Verification items for the finished model (mm, model axes). Face numbers are marked on the shaded views. A direction names the side the tool comes from. Coordinates: 2 decimals unless noted, no trailing zeros. Order: outer loops, then holes, each group sorted by start corner. A loop starts at its lowest first (then second) coordinate and runs counter-clockwise, first axis right, second up. Notation, with made-up numbers: M 81.5,4 L 94.5,4 A25 cw 94.5,20 Z; hole C 42.25,-35.75 d6. An arc over 180 degrees is marked long. Return JSON: item names as keys, results as strings. Group by question number.
1. Gauge pin test, flat end, axial feed: pin 1 (8 mm diameter, centred on x = 25, z = 15, fed in from +Y). Record the tip position at first contact, or that the pin passes through.
2. Mould release check, pull along Z, two halves, no side actions. Record for the marked faces 1, 2, 3 and 4: +Z half, -Z half, draft (parallel to the pull), parting line (faces both ways), or undercut.
3. Section check D-D, the plane x = 33. Record the cut outline in (y, z), plus the area to 3 significant figures.
4. Section check A-A, the plane z = 15. Record the cut outline in (x, y), plus the area to 4 significant figures.
5. Section check C-C, the plane y = 124.5. Record the cut outline in (x, z).
6. Set-up check for the marked faces 5 and 6: record each of +Z, -Z, +X, -X, +Y, -Y from which the full face is reachable in a straight line by a thin tool's end or side.
7. Section check B-B, the plane y = 66. Record the cut outline in (x, z).
8. Material ranges on line 1 along X through (y, z) = (-1, 15); line 2 along Z through (x, y) = (12, 105); line 3 along Y through (x, z) = (4.5, 16.5), recorded low to high.
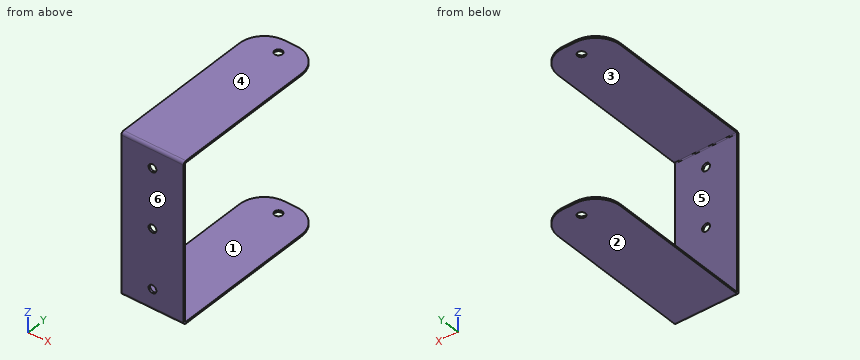
```python
from build123d import *

# Parameters (mm, degrees)
SKETCH1_W                    = 50
SKETCH1_H                    = 125
BASE_FLANGE1_DEPTH           = 1.5
EDGE_FLANGE1_STRIP_W         = 7.5
EDGE_FLANGE1_STRIP_H         = 1.5
EDGE_FLANGE1_STRIP_CUT_DEPTH = 50
EDGE_FLANGE1_DEPTH           = 50
SKETCH9_R                    = 3.15
CUT_EXTRUDE1_DEPTH           = 176
EDGE_FLANGE2_STRIP_W         = 7.5
EDGE_FLANGE2_STRIP_H         = 1.5
EDGE_FLANGE2_STRIP_CUT_DEPTH = 50
EDGE_FLANGE2_DEPTH           = 50
CUT_EXTRUDE2_START           = -10
SKETCH13_R                   = 3.15
CUT_EXTRUDE2_DEPTH           = 10
FILLET1_R                    = 20
SKETCH14_R                   = 3.15
CUT_EXTRUDE3_DEPTH           = 10


# Sheet-metal steps are written as plain solids
with BuildPart() as part:
    # Sketch1 → Base-Flange1 (new body)
    with BuildSketch(Plane(origin=(0, 0, 0), x_dir=(1, 0, 0), z_dir=(0, 1, 0))):
        with Locations((25, -62.5)):
            Rectangle(SKETCH1_W, SKETCH1_H)
    extrude(amount=-BASE_FLANGE1_DEPTH)

    # Edge-Flange1 strip (across the edge) → Edge-Flange1 strip cut (cut)
    with BuildSketch(Plane(origin=(0, 0, 125), x_dir=(0, 0, -1), z_dir=(1, 0, 0))):
        with Locations((-3, -0.75)):
            Rectangle(EDGE_FLANGE1_STRIP_W, EDGE_FLANGE1_STRIP_H)
    extrude(amount=EDGE_FLANGE1_STRIP_CUT_DEPTH, mode=Mode.SUBTRACT)

    # Edge-Flange1 section (across the edge) → Edge-Flange1 (add)
    with BuildSketch(Plane(origin=(0, 0, 125), x_dir=(0, 0, -1), z_dir=(1, 0, 0))):
        with BuildLine():
            Line((-1.5, 0.75), (-1.5, 136.5))
            Line((-1.5, 136.5), (0, 136.5))
            Line((0, 136.5), (0, 0.75))
            ThreePointArc((0, 0.75), (0.219669914, 0.219669914), (0.75, 0))
            Line((0.75, 0), (0.75, -1.5))
            ThreePointArc((0.75, -1.5), (-0.840990258, -0.840990258), (-1.5, 0.75))
        make_face()
    extrude(amount=EDGE_FLANGE1_DEPTH)

    # Sketch9 → Cut-Extrude1 (cut)
    with BuildSketch(Plane.XY.offset(126.5)):
        with Locations((25, 124.5)):
            Circle(SKETCH9_R)
    extrude(amount=-CUT_EXTRUDE1_DEPTH, mode=Mode.SUBTRACT)

    # Edge-Flange2 strip (across the edge) → Edge-Flange2 strip cut (cut)
    with BuildSketch(Plane.ZY.offset(-50)):
        with Locations((-3, -0.75)):
            Rectangle(EDGE_FLANGE2_STRIP_W, EDGE_FLANGE2_STRIP_H)
    extrude(amount=EDGE_FLANGE2_STRIP_CUT_DEPTH, mode=Mode.SUBTRACT)

    # Edge-Flange2 section (across the edge) → Edge-Flange2 (add)
    with BuildSketch(Plane.ZY.offset(-50)):
        with BuildLine():
            Line((-1.5, 0.75), (-1.5, 136.5))
            Line((-1.5, 136.5), (0, 136.5))
            Line((0, 136.5), (0, 0.75))
            ThreePointArc((0, 0.75), (0.219669914, 0.219669914), (0.75, 0))
            Line((0.75, 0), (0.75, -1.5))
            ThreePointArc((0.75, -1.5), (-0.840990258, -0.840990258), (-1.5, 0.75))
        make_face()
    extrude(amount=EDGE_FLANGE2_DEPTH)

    # Sketch13 → Cut-Extrude2 (cut)
    with BuildSketch(Plane(origin=(0, 0, -1.5), x_dir=(-1, 0, 0), z_dir=(0, 0, -1)).offset(CUT_EXTRUDE2_START)):
        with Locations(Location((-25, 124.5, 0), (0, 0, 180))):
            Circle(SKETCH13_R)
    extrude(amount=CUT_EXTRUDE2_DEPTH, mode=Mode.SUBTRACT)

    # Fillet1
    fillet1_edges = [part.edges().sort_by_distance(p)[0] for p in [
        (0, 136.5, 125.75),
        (50, 136.5, 125.75),
        (50, 136.5, -0.75),
        (0, 136.5, -0.75),
    ]]
    fillet(fillet1_edges, radius=FILLET1_R)

    # Sketch14 → Cut-Extrude3 (cut)
    with BuildSketch(Plane(origin=(0, 0, 0), x_dir=(1, 0, 0), z_dir=(0, 1, 0))):
        with Locations(Location((25, -15, 0), (0, 0, 270))):
            Circle(SKETCH14_R)
        with Locations(Location((25, -62.5, 0), (0, 0, 270))):
            Circle(SKETCH14_R)
        with Locations(Location((25, -110, 0), (0, 0, 270))):
            Circle(SKETCH14_R)
    extrude(amount=-CUT_EXTRUDE3_DEPTH, mode=Mode.SUBTRACT)


solid = part.part
```
Answers follow:
{
 "1": {"pin 1": "y = 0"},
 "2": {"face 1": "undercut", "face 2": "-Z half", "face 3": "undercut", "face 4": "+Z half"},
 "3": {"outline": "M -1.5,0.75 A2.25 ccw 0.75,-1.5 L 136.27,-1.5 L 136.27,0 L 0.75,0 A0.75 cw 0,0.75 L 0,124.25 A0.75 cw 0.75,125 L 136.27,125 L 136.27,126.5 L 0.75,126.5 A2.25 ccw -1.5,124.25 Z", "area": "599 mm^2"},
 "4": {"outline": "M 0,-1.5 L 21.85,-1.5 L 21.85,0 L 0,0 Z; M 28.15,-1.5 L 50,-1.5 L 50,0 L 28.15,0 Z", "area": "65.55 mm^2"},
 "5": {"outline": "M 1.67,-1.5 L 21.85,-1.5 L 21.85,0 L 1.67,0 Z; M 1.67,125 L 21.85,125 L 21.85,126.5 L 1.67,126.5 Z; M 28.15,-1.5 L 48.33,-1.5 L 48.33,0 L 28.15,0 Z; M 28.15,125 L 48.33,125 L 48.33,126.5 L 28.15,126.5 Z"},
 "6": {"face 5": "+X, -X, +Y", "face 6": "+Z, -Z, +X, -X, -Y"},
 "7": {"outline": "M 0,-1.5 L 50,-1.5 L 50,0 L 0,0 Z; M 0,125 L 50,125 L 50,126.5 L 0,126.5 Z"},
 "8": {"line 1": "0 to 21.85, 28.15 to 50", "line 2": "-1.5 to 0, 125 to 126.5", "line 3": "-1.5 to 0"}
}
